```python
from build123d import *

# Parameters (mm, degrees)
SKETCH1_R           = 2.5
BOSS_EXTRUDE1_DEPTH = 100
SKETCH2_R           = 2.5
CUT_EXTRUDE1_DEPTH  = 1


with BuildPart() as part:
    # Sketch1 → Boss-Extrude1 (new body)
    with BuildSketch(Plane(origin=(0, 0, 0), x_dir=(1, 0, 0), z_dir=(0, 1, 0))):
        with BuildLine():
            Line((-5.357713917, -5.679481981), (-3.657713917, -5.679481981))
            ThreePointArc((-3.657713917, -5.679481981), (-3.5516479, -5.635547998), (-3.507713917, -5.529481981))
            Line((-3.507713917, -5.529481981), (-3.507713917, -2.093297468))
            ThreePointArc((-3.507713917, -2.093297468), (-3.415514871, -1.954881249), (-3.252259921, -1.98662294))
            Line((-3.252259921, -1.98662294), (0.53858238, -5.734091759))
            Line((0.53858238, -5.734091759), (0.53858238, -11.624872203))
            Line((0.53858238, -11.624872203), (-3.252259921, -15.372341022))
            ThreePointArc((-3.252259921, -15.372341022), (-3.415514871, -15.404082713), (-3.507713917, -15.265666494))
            Line((-3.507713917, -15.265666494), (-3.507713917, -11.829481981))
            ThreePointArc((-3.507713917, -11.829481981), (-3.5516479, -11.723415964), (-3.657713917, -11.679481981))
            Line((-3.657713917, -11.679481981), (-5.357713917, -11.679481981))
            ThreePointArc((-5.357713917, -11.679481981), (-5.463779934, -11.723415964), (-5.507713917, -11.829481981))
            Line((-5.507713917, -11.829481981), (-5.507713917, -18.329481981))
            ThreePointArc((-5.507713917, -18.329481981), (-5.40520129, -18.576969354), (-5.157713917, -18.679481981))
            Line((-5.157713917, -18.679481981), (1.342286083, -18.679481981))
            ThreePointArc((1.342286083, -18.679481981), (1.4483521, -18.635547998), (1.492286083, -18.529481981))
            Line((1.492286083, -18.529481981), (1.492286083, -16.829481981))
            ThreePointArc((1.492286083, -16.829481981), (1.4483521, -16.723415964), (1.342286083, -16.679481981))
            Line((1.342286083, -16.679481981), (-2.075798714, -16.679481981))
            ThreePointArc((-2.075798714, -16.679481981), (-2.214545208, -16.586485581), (-2.181252709, -16.422807453))
            Line((-2.181252709, -16.422807453), (1.605398289, -12.679481981))
            Line((1.605398289, -12.679481981), (7.379173877, -12.679481981))
            Line((7.379173877, -12.679481981), (11.165824876, -16.422807453))
            ThreePointArc((11.165824876, -16.422807453), (11.199117374, -16.586485581), (11.06037088, -16.679481981))
            Line((11.06037088, -16.679481981), (7.642286083, -16.679481981))
            ThreePointArc((7.642286083, -16.679481981), (7.536220066, -16.723415964), (7.492286083, -16.829481981))
            Line((7.492286083, -16.829481981), (7.492286083, -18.529481981))
            ThreePointArc((7.492286083, -18.529481981), (7.536220066, -18.635547998), (7.642286083, -18.679481981))
            Line((7.642286083, -18.679481981), (14.142286083, -18.679481981))
            ThreePointArc((14.142286083, -18.679481981), (14.389773457, -18.576969354), (14.492286083, -18.329481981))
            Line((14.492286083, -18.329481981), (14.492286083, -11.829481981))
            ThreePointArc((14.492286083, -11.829481981), (14.4483521, -11.723415964), (14.342286083, -11.679481981))
            Line((14.342286083, -11.679481981), (12.642286083, -11.679481981))
            ThreePointArc((12.642286083, -11.679481981), (12.536220066, -11.723415964), (12.492286083, -11.829481981))
            Line((12.492286083, -11.829481981), (12.492286083, -15.265666494))
            ThreePointArc((12.492286083, -15.265666494), (12.400087038, -15.404082713), (12.236832088, -15.372341022))
            Line((12.236832088, -15.372341022), (8.445989787, -11.624872203))
            Line((8.445989787, -11.624872203), (8.445989787, -5.734091759))
            Line((8.445989787, -5.734091759), (12.236832088, -1.98662294))
            ThreePointArc((12.236832088, -1.98662294), (12.400087038, -1.954881249), (12.492286083, -2.093297468))
            Line((12.492286083, -2.093297468), (12.492286083, -5.529481981))
            ThreePointArc((12.492286083, -5.529481981), (12.536220066, -5.635547998), (12.642286083, -5.679481981))
            Line((12.642286083, -5.679481981), (14.342286083, -5.679481981))
            ThreePointArc((14.342286083, -5.679481981), (14.4483521, -5.635547998), (14.492286083, -5.529481981))
            Line((14.492286083, -5.529481981), (14.492286083, 0.970518019))
            ThreePointArc((14.492286083, 0.970518019), (14.389773457, 1.218005392), (14.142286083, 1.320518019))
            Line((14.142286083, 1.320518019), (7.642286083, 1.320518019))
            ThreePointArc((7.642286083, 1.320518019), (7.536220066, 1.276584036), (7.492286083, 1.170518019))
            Line((7.492286083, 1.170518019), (7.492286083, -0.529481981))
            ThreePointArc((7.492286083, -0.529481981), (7.536220066, -0.635547998), (7.642286083, -0.679481981))
            Line((7.642286083, -0.679481981), (11.06037088, -0.679481981))
            ThreePointArc((11.06037088, -0.679481981), (11.199117374, -0.772478381), (11.165824876, -0.936156509))
            Line((11.165824876, -0.936156509), (7.379173877, -4.679481981))
            Line((7.379173877, -4.679481981), (1.605398289, -4.679481981))
            Line((1.605398289, -4.679481981), (-2.181252709, -0.936156509))
            ThreePointArc((-2.181252709, -0.936156509), (-2.214545208, -0.772478381), (-2.075798714, -0.679481981))
            Line((-2.075798714, -0.679481981), (1.342286083, -0.679481981))
            ThreePointArc((1.342286083, -0.679481981), (1.4483521, -0.635547998), (1.492286083, -0.529481981))
            Line((1.492286083, -0.529481981), (1.492286083, 1.170518019))
            ThreePointArc((1.492286083, 1.170518019), (1.4483521, 1.276584036), (1.342286083, 1.320518019))
            Line((1.342286083, 1.320518019), (-5.157713917, 1.320518019))
            ThreePointArc((-5.157713917, 1.320518019), (-5.40520129, 1.218005392), (-5.507713917, 0.970518019))
            Line((-5.507713917, 0.970518019), (-5.507713917, -5.529481981))
            ThreePointArc((-5.507713917, -5.529481981), (-5.463779934, -5.635547998), (-5.357713917, -5.679481981))
        make_face()
        with Locations(Location((4.492286083, -8.679481981, 0), (0, 0, 270))):
            Circle(SKETCH1_R, mode=Mode.SUBTRACT)
    extrude(amount=BOSS_EXTRUDE1_DEPTH)

    # Sketch2 → Cut-Extrude1 (cut)
    with BuildSketch(Plane.XY.offset(12.679481981)):
        with Locations((4.492286083, 53.418394615)):
            Circle(SKETCH2_R)
        with Locations((4.492286083, 93.418394615)):
            Circle(SKETCH2_R)
    extrude(amount=-CUT_EXTRUDE1_DEPTH, mode=Mode.SUBTRACT)


solid = part.part
```
Design review of the part built by this model. Coordinates are the model's own, in mm. A direction names the side the tool comes from. Give positions to 0.01 mm unless a question says otherwise; leave off trailing zeros. Order: outer loops, then holes, each group sorted by start corner. A loop starts at its lowest first (then second) coordinate and runs counter-clockwise, first axis right, second up. Notation, with made-up numbers: (1, 14.25) - (57, 14.25) arc R27 cw to (57, 39.25) - close; hole circle Ø8 at (47, -18.75). An arc over 180 degrees is marked (long way). Use a Markdown table: item, result. Add a question column.
(1) Add section A-A on z = 8. Give the boundary of the cut face in (x, y), then the cut area to 3 significant figures.
(2) Machinability: for faces 4 (the face through (4, 53, 11.679)), 5 (the face through (-3.508, 49, 14)), 6 (the face through (4, 49, 12.679)), which of the approach directions +Z, -Z, +X, -X, +Y, -Y give a long, thin tool a straight path to every point of the face, cutting with its end or side? Answer none if there is none.
(3) Wall thickness on probe 1 along X at (y, z) = (55, 12); probe 2 along X at (y, z) = (53.5, 15); probe 3 along X at (y, z) = (85, 12): over which ranges is each line inside the solid? List them lowest first. Write a range as [from, to].
(4) Mouldability with a two-part tool opening along X and no side actions: class faces 1 (the face through (8.446, 49, 9)), 2 (the face through (-0.314, 49.3, 14.577)), 3 (the face through (0.539, 49, 9)) as +X half, -X half, draft (parallel to the pull), parting line (faces both ways), or undercut.
(5) Clearance check with flat-ended pins moving along their axes: P1, Ø12, axis at x = 7.5, y = 73, coming from the +Z side; P2, Ø1.7, axis at x = 5.5, y = 39.5, coming from the +Z side; P3, Ø3, axis at x = 4.5, y = 39.5, coming from the -Z side. State where each tip first meets the part, or that it passes through.
Report:
| question | item | result |
|---|---|---|
| 1 | outline | (0.54, 0) - (2.09, 0) - (2.09, 100) - (0.54, 100) - close; (6.9, 0) - (8.45, 0) - (8.45, 100) - (6.9, 100) - close |
| 1 | area | 310 mm² |
| 2 | face 4 | +Z |
| 2 | face 5 | +Y, -Y |
| 2 | face 6 | +Z, +Y, -Y |
| 3 | probe 1 | x = [-5.51, -3.51], [0.16, 2.56], [6.43, 8.83], [12.49, 14.49] |
| 3 | probe 2 | x = [-5.51, -3.51], [-2.88, -0.74], [9.73, 11.86], [12.49, 14.49] |
| 3 | probe 3 | x = [-5.51, -3.51], [0.16, 8.83], [12.49, 14.49] |
| 4 | face 1 | +X half |
| 4 | face 2 | undercut |
| 4 | face 3 | -X half |
| 5 | P1 | stops at z = 18.68 |
| 5 | P2 | stops at z = 12.68 |
| 5 | P3 | stops at z = 4.68 |
